```python
from build123d import *

# Parameters (mm, degrees)
F2_R     = 5
F3_SIZE  = 6.49999
F4_SIZE2 = 1
F4_SIZE  = 2.7474774195


# Not quite as in the source:
# - a fillet or chamfer is up to 0.001 mm smaller than in the source, because OpenCascade refuses the exact size


with BuildPart() as f1:
    # F0 (on Front) → F1 (revolve)
    with BuildSketch(Plane.XZ):
        Polygon((-18, 0), (0, 0), (0, 71), (-24.5, 71), (-24.5, 56), (-18, 56), (-18, 41), (-24.5, 41), (-24.5, 38), (-18, 38), align=None)
    revolve(axis=Axis((0, 0, 35.5), (0, 0, 1)))

    # F2
    f2_edges = [f1.edges().sort_by_distance(p)[0] for p in [
        (24.5, 0, 56),
        (24.5, 0, 71),
    ]]
    fillet(f2_edges, radius=F2_R)

    # F3 (size 6.5 in the source; OpenCascade refuses exactly that, so slightly less here)
    f3_edges = [f1.edges().sort_by_distance(p)[0] for p in [
        (18, 0, 41),
    ]]
    chamfer(f3_edges, length=F3_SIZE)

    # F4
    f4_edges = [f1.edges().sort_by_distance(p)[0] for p in [
        (18, 0, 0),
    ]]
    f4_side = f1.faces().sort_by_distance((18, 0, 19))[0]
    chamfer(f4_edges, length=F4_SIZE, length2=F4_SIZE2, reference=f4_side)


solid = f1.part
```
For this review, take the finished solid that the model builds, in its own axes (mm). A direction names the side the tool comes from. Coordinates: 2 decimals unless noted, no trailing zeros. Loops run counter-clockwise (first coordinate to the right, second up) from the corner with the lowest first, then second, coordinate; pieces in that order, holes last.
1. For line 1 (Z direction, x = -17, y = 6.5); line 2 (Z direction, x = 18.5, y = 9.5); line 3 (Y direction, x = 12.5, z = 3.5), list the stretches that pass through material, from the lowest coordinate up.
2. Add section D-D, the plane z = 31.5. Give the boundary of the cut face in (x, y), then the cut area to 3 significant figures.
3. Mouldability with a two-part tool opening along Z and no side actions: class faces 4 (the flat face through (0, 0, 0)), 5 (the cylindrical face through (2.343, -17.847, 20.127)), 6 (the conical face through (14.6, 11.2, 47.1)) as +Z half, -Z half, draft (parallel to the pull), parting line (faces both ways), or undercut.
4. Insertion check: P1, Ø5, axis at x = -9.5, z = 46, coming from the +Y side; P2, Ø5, axis at y = 11.5, z = 59.5, coming from the +X side; P3, Ø6, axis at x = -0.5, z = 30.5, coming from the -Y side. Each pin has a flat end and moves straight along its axis. Give the tip position at first contact, or say it passes through.
5. For faces 1 (the cylindrical face through (-13.17, -20.66, 39.48)), 2 (the flat face through (13, -13, 38)), 3 (the cylindrical face through (2.343, -17.847, 51.69)), list the 3-axis set-ups (+Z, -Z, +X, -X, +Y, -Y) from which the entire face can be reached by the end or side of a thin tool; tool diameter is ignored.
6. Add section C-C, the plane z = 65. Give the boundary of the cut face in (x, y), then the cut area to 3 significant figures.
Result:
1. line 1: z = 38 to 47.3, 56 to 71
1. line 2: z = 38 to 44.7, 56.17 to 70.83
1. line 3: y = -12.95 to 12.95
2. outline: circle Ø36 at (0, 0)
2. area: 1,020 mm2
3. face 4: -Z half
3. face 5: draft
3. face 6: undercut
4. P1: stops at y = 20.07
4. P2: stops at x = 22.68
4. P3: stops at y = -18
5. face 1: +Z, -Z
5. face 2: -Z
5. face 3: none
6. outline: circle Ø49 at (0, 0)
6. area: 1,890 mm2
